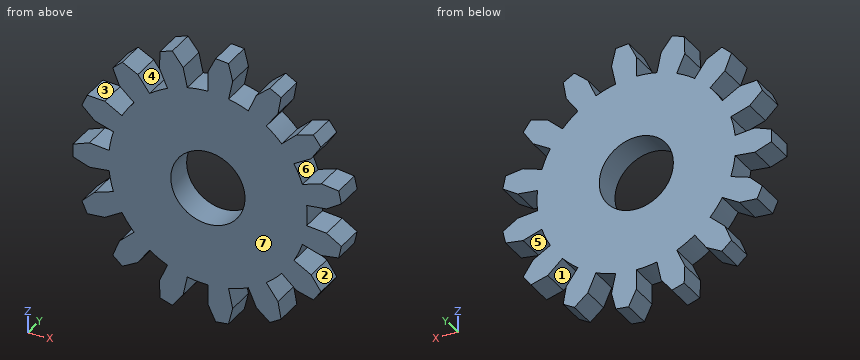
Autodesk Inventor part; units mm, degrees
ref_plane "YZ Plane" through (0, 0, 0) normal (1, 0, 0) x (0, 1, 0)
ref_plane "XZ Plane" through (0, 0, 0) normal (0, 1, 0) x (-1, 0, 0)
ref_plane "XY Plane" through (0, 0, 0) normal (0, 0, 1) x (1, 0, 0)
sketch "スケッチ1" plane through (0, 0, 0) normal (0, 1, 0) x (-1, 0, 0)
  circle A0 centre (0, 0) radius 22.5 construction
  circle A1 centre (0, 0) radius 25.5 construction
  line L0 (25.5, 1.2181) -> (25.5, -1.2181)
  line L1 (25.5, 1.2181) -> (22.3764, 2.355)
  line L2 (25.5, -1.2181) -> (22.3764, -2.355)
  line L3 (35.7, 0) -> (-35.7, 0)
  circle A2 centre (0, 0) radius 18.75
  line L4 (22.3764, -2.355) -> (18.647, -1.9625)
  line L5 (22.3764, 2.355) -> (18.647, 1.9625)
  line L6 (19.484, 11.2527) -> (16.2367, 9.3773)
  line L7 (22.8, 11.4846) -> (19.484, 11.2527)
  line L8 (22.8, 11.4846) -> (23.7909, 9.259)
  line L9 (23.7909, 9.259) -> (21.3997, 6.9499)
  line L10 (21.3997, 6.9499) -> (17.8331, 5.7916)
  line L11 (13.2226, 18.2047) -> (11.0189, 15.1706)
  line L12 (16.1576, 19.7653) -> (13.2226, 18.2047)
  line L13 (16.1576, 19.7653) -> (17.9681, 18.1351)
  line L14 (17.9681, 18.1351) -> (16.7229, 15.0531)
  line L15 (16.7229, 15.0531) -> (13.9357, 12.5443)
  line L16 (4.675, 22.009) -> (3.8958, 18.3408)
  line L17 (6.7214, 24.6284) -> (4.675, 22.009)
  line L18 (6.7214, 24.6284) -> (9.0384, 23.8755)
  line L19 (9.0384, 23.8755) -> (9.1544, 20.5535)
  line L20 (9.1544, 20.5535) -> (7.6287, 17.1279)
  line L21 (-4.6811, 22.0077) -> (-3.9009, 18.3397)
  line L22 (-3.8769, 25.233) -> (-4.6811, 22.0077)
  line L23 (-3.8769, 25.233) -> (-1.454, 25.4876)
  line L24 (-1.454, 25.4876) -> (0.0031, 22.5)
  line L25 (0.0031, 22.5) -> (0.0026, 18.75)
  line L26 (-13.2277, 18.201) -> (-11.0231, 15.1675)
  line L27 (-13.8049, 21.4746) -> (-13.2277, 18.201)
  line L28 (-13.8049, 21.4746) -> (-11.6951, 22.6927)
  line L29 (-11.6951, 22.6927) -> (-9.1487, 20.556)
  line L30 (-9.1487, 20.556) -> (-7.6239, 17.13)
  line L31 (-19.4871, 11.2473) -> (-16.2393, 9.3727)
  line L32 (-21.3459, 14.0031) -> (-19.4871, 11.2473)
  line L33 (-21.3459, 14.0031) -> (-19.9139, 15.974)
  line L34 (-19.9139, 15.974) -> (-16.7187, 15.0578)
  line L35 (-16.7187, 15.0578) -> (-13.9322, 12.5481)
  line L36 (-22.3771, 2.3488) -> (-18.6476, 1.9573)
  line L37 (-25.196, 4.1103) -> (-22.3771, 2.3488)
  line L38 (-25.196, 4.1103) -> (-24.6895, 6.4932)
  line L39 (-24.6895, 6.4932) -> (-21.3978, 6.9559)
  line L40 (-21.3978, 6.9559) -> (-17.8315, 5.7965)
  line L41 (-21.3978, -6.9559) -> (-17.8315, -5.7965)
  line L42 (-24.6895, -6.4932) -> (-21.3978, -6.9559)
  line L43 (-24.6895, -6.4932) -> (-25.196, -4.1103)
  line L44 (-25.196, -4.1103) -> (-22.3771, -2.3488)
  line L45 (-22.3771, -2.3488) -> (-18.6476, -1.9573)
  line L46 (-16.7187, -15.0578) -> (-13.9322, -12.5481)
  line L47 (-19.9139, -15.974) -> (-16.7187, -15.0578)
  line L48 (-19.9139, -15.974) -> (-21.3459, -14.0031)
  line L49 (-21.3459, -14.0031) -> (-19.4871, -11.2473)
  line L50 (-19.4871, -11.2473) -> (-16.2393, -9.3727)
  line L51 (-9.1487, -20.556) -> (-7.6239, -17.13)
  line L52 (-11.6951, -22.6927) -> (-9.1487, -20.556)
  line L53 (-11.6951, -22.6927) -> (-13.8049, -21.4746)
  line L54 (-13.8049, -21.4746) -> (-13.2277, -18.201)
  line L55 (-13.2277, -18.201) -> (-11.0231, -15.1675)
  line L56 (0.0031, -22.5) -> (0.0026, -18.75)
  line L57 (-1.454, -25.4876) -> (0.0031, -22.5)
  line L58 (-1.454, -25.4876) -> (-3.8769, -25.233)
  line L59 (-3.8769, -25.233) -> (-4.6811, -22.0077)
  line L60 (-4.6811, -22.0077) -> (-3.9009, -18.3397)
  line L61 (9.1544, -20.5535) -> (7.6287, -17.1279)
  line L62 (9.0384, -23.8755) -> (9.1544, -20.5535)
  line L63 (9.0384, -23.8755) -> (6.7214, -24.6284)
  line L64 (6.7214, -24.6284) -> (4.675, -22.009)
  line L65 (4.675, -22.009) -> (3.8958, -18.3408)
  line L66 (16.7229, -15.0531) -> (13.9357, -12.5443)
  line L67 (17.9681, -18.1351) -> (16.7229, -15.0531)
  line L68 (17.9681, -18.1351) -> (16.1576, -19.7653)
  line L69 (16.1576, -19.7653) -> (13.2226, -18.2047)
  line L70 (13.2226, -18.2047) -> (11.0189, -15.1706)
  line L71 (21.3997, -6.9499) -> (17.8331, -5.7916)
  line L72 (23.7909, -9.259) -> (21.3997, -6.9499)
  line L73 (23.7909, -9.259) -> (22.8, -11.4846)
  line L74 (22.8, -11.4846) -> (19.484, -11.2527)
  line L75 (19.484, -11.2527) -> (16.2367, -9.3773)
  circle A3 centre (0, 0) radius 7
  point P0 (25.5, 0)
  point P1 (23.2954, 10.3718)
  point P2 (17.0628, 18.9502)
  point P3 (7.8799, 24.2519)
  point P4 (-2.6655, 25.3603)
  point P5 (-12.75, 22.0836)
  point P6 (-20.6299, 14.9885)
  point P7 (-24.9428, 5.3017)
  point P8 (-24.9428, -5.3017)
  point P9 (-20.6299, -14.9885)
  point P10 (-12.75, -22.0836)
  point P11 (-2.6655, -25.3603)
  point P12 (7.8799, -24.2519)
  point P13 (17.0628, -18.9502)
  point P14 (23.2954, -10.3718)
  point P15 (17.8331, 5.7916)
  point P16 (16.2367, 9.3773)
  point P17 (13.9357, 12.5443)
  point P18 (11.0189, 15.1706)
  point P19 (7.6287, 17.1279)
  point P20 (3.8958, 18.3408)
  point P21 (0.0026, 18.75)
  point P22 (-3.9009, 18.3397)
  point P23 (-7.6239, 17.13)
  point P24 (-11.0231, 15.1675)
  point P25 (-13.9322, 12.5481)
  point P26 (-16.2393, 9.3727)
  point P27 (-17.8315, 5.7965)
  point P28 (-18.6476, 1.9573)
  point P29 (-18.6476, -1.9573)
  point P30 (-17.8315, -5.7965)
  point P31 (-16.2393, -9.3727)
  point P32 (-13.9322, -12.5481)
  point P33 (-11.0231, -15.1675)
  point P34 (-7.6239, -17.13)
  point P35 (-3.9009, -18.3397)
  point P36 (0.0026, -18.75)
  point P37 (3.8958, -18.3408)
  point P38 (7.6287, -17.1279)
  point P39 (11.0189, -15.1706)
  point P40 (13.9357, -12.5443)
  point P41 (16.2367, -9.3773)
  point P42 (17.8331, -5.7916)
  dimension "d5" = 37.5
  dimension "d0" = 45
  dimension "d1" = 51
  dimension "d3" = 20
  dimension "d4" = 20
  dimension "d14" = 4.71
  dimension "d18" = 360
  dimension "d23" = 14
extrude "押し出し1" add sketch "スケッチ1" along normal blind 5.5 contours L0 L3 A2 L5 L1 | L0 L2 L4 A2 L3 | A2 L3 A3 | L3 A3 A2 | A2 L6 L7 L8 L9 L10 | L71 L72 L73 L74 L75 A2 | A2 L11 L12 L13 L14 L15 | L36 L37 L38 L39 L40 A2 | A2 L41 L42 L43 L44 L45 | L66 L67 L68 L69 L70 A2 | A2 L16 L17 L18 L19 L20 | L31 L32 L33 L34 L35 A2 | A2 L46 L47 L48 L49 L50 | L61 L62 L63 L64 L65 A2 | A2 L21 L22 L23 L24 L25 | L26 L27 L28 L29 L30 A2 | A2 L51 L52 L53 L54 L55 | L56 L57 L58 L59 L60 A2
properties part number "M3_15_hole_small" material "木材 (カエデ材)"
Work out the finished part from the listing and answer in its coordinate system (mm). Face numbers are marked on the shaded views. A direction names the side the tool comes from. Round coordinates to 2 decimals unless told otherwise and drop trailing zeros. Write each loop counter-clockwise with the first axis right and the second up, starting at its lowest first coordinate (ties: lowest second). Pieces come first, ordered by that corner, then holes. Notation, with made-up numbers: (-32, 41.5) - (-2, 41.5) arc R37 ccw to (-2, 79.5) - close; hole circle Ø8 at (50, 84). An arc over 180 degrees is marked (long way). Answer in a Markdown table with one row per item. Add a question column.
1. Given pin 1 (8.5 mm diameter, centred on x = 0, z = 0, fed in from +Y); pin 2 (1.5 mm diameter, centred on y = 1, z = 18, fed in from -X); pin 3 (3 mm diameter, centred on y = 3, z = -20, fed in from -X); pin 4 (1.5 mm diameter, centred on x = -2, y = 1, fed in from +Z), each flat-ended and moving along its own axis, determine where each tip first touches the part or whether it passes through.
2. A cutting plane is placed at A-A, the plane z = 0. Determine the outline of the cut face in (x, y).
3. The mould has two halves that part along Z. Classify the marked faces 4, 5, 6 and 7: +Z half, -Z half, draft (parallel to the pull), parting line (faces both ways), or undercut.
4. For the marked faces 1, 2 and 3, determine the directions among +Z, -Z, +X, -X, +Y, -Y from which every point of the face is accessible in a straight line to the end or side of a thin tool.
5. Find the intervals of material crossed by line 1 along X through (y, z) = (3.3, 0); line 2 along Z through (x, y) = (17, 0.85); line 3 along X through (y, z) = (4.4, -20.5), in increasing order. Write a range as from..to.
Worked out:
| question | item | result |
|---|---|---|
| 1 | pin 1 | through |
| 1 | pin 2 | x = -17.97 |
| 1 | pin 3 | x = -17.56 |
| 1 | pin 4 | z = 18.71 |
| 2 | outline | (-25.5, 0) - (-7, 0) - (-7, 5.5) - (-25.5, 5.5) - close; (7, 0) - (18.75, 0) - (18.75, 5.5) - (7, 5.5) - close |
| 3 | face 4 | +Z half |
| 3 | face 5 | undercut |
| 3 | face 6 | undercut |
| 3 | face 7 | draft |
| 4 | face 1 | -Z, +Y, -Y |
| 4 | face 2 | +X, +Y, -Y |
| 4 | face 3 | +Z, +Y, -Y |
| 5 | line 1 | -25.5..-7, 7..18.75 |
| 5 | line 2 | -15.14..-9.81, -7.91..7.91, 9.81..15.14 |
| 5 | line 3 | -9.13..-4.35, 0..4.36, 9.12..13.63 |
